For this review, take the finished solid that the model builds, in its own axes (mm). Face numbers are marked on the shaded views. A direction names the side the tool comes from. Give positions to 0.01 mm unless a question says otherwise; leave off trailing zeros. Order: outer loops, then holes, each group sorted by start corner. A loop starts at its lowest first (then second) coordinate and runs counter-clockwise, first axis right, second up.
Item 1: The part is to be moulded in two halves that separate along Y. For the marked faces 1, 2 and 3, say which applies: released by +Y, released by -Y, zero draft, split by the parting line, or undercut.
Item 2: Consider section A-A (z = -58). Give the number of separate pieces and of enclosed holes in the cut face, plus the area to 3 significant figures.
Item 3: Machinability: for the marked faces 4, 5 and 6, which of the approach directions +Z, -Z, +X, -X, +Y, -Y give a long, thin tool a straight path to every point of the face, cutting with its end or side? Answer none if there is none.
Item 4: Consider section B-B (x = 5). Give the boundary of the cut face in (y, z).
Item 5: For probe 1 along Y at (x, z) = (1.5, -26.5); probe 2 along Y at (x, z) = (-23, -48); probe 3 along Y at (x, z) = (18, -7), list the stretches that pass through material, from the lowest coordinate up.
Item 6: For P1, Ø1.2, axis at y = -24.5, z = -34, coming from the -X side; P2, Ø3, axis at y = -7, z = -25.5, coming from the -X side; P3, Ø2.5, axis at x = 13.97, y = 52.14, coming from the -Z side; P4, Ø4, axis at x = 37, z = -62, coming from the -Y side, all flat-tipped, find the tip position at first contact; note any pin that passes through.
```python
from build123d import *

# Parameters (mm, degrees)
SKETCH1_R                                     = 63.5
BOSS_EXTRUDE1_DEPTH                           = 6.35
BOSS_EXTRUDE2_START                           = 19.5
SKETCH1_3_R                                   = 44.45
BOSS_EXTRUDE2_DEPTH                           = 101.6
CUT_EXTRUDE1_DEPTH                            = 136.598893801
FILLET1_R                                     = 3.75
CUT_EXTRUDE2_DEPTH                            = 5
SKETCH4_R                                     = 63.5
SKETCH4_R_2                                   = 44.45
BOSS_EXTRUDE3_DEPTH                           = 15.4
CSK_FOR_8_FLAT_HEAD_MACHINE_SCREW1_AT_2_COUNT = 2
CSK_FOR_8_FLAT_HEAD_MACHINE_SCREW1_AT_2_PITCH = 53.975
CSK_FOR_8_FLAT_HEAD_MACHINE_SCREW1_AT_3_COUNT = 2
CSK_FOR_8_FLAT_HEAD_MACHINE_SCREW1_AT_3_PITCH = 93.487442339
CSK_FOR_8_FLAT_HEAD_MACHINE_SCREW1_AT_4_COUNT = 2
CSK_FOR_8_FLAT_HEAD_MACHINE_SCREW1_AT_4_PITCH = 107.95
CSK_FOR_8_FLAT_HEAD_MACHINE_SCREW1_AT_5_COUNT = 2
CSK_FOR_8_FLAT_HEAD_MACHINE_SCREW1_AT_5_PITCH = 93.487442339
CSK_FOR_8_FLAT_HEAD_MACHINE_SCREW1_AT_6_COUNT = 2
CSK_FOR_8_FLAT_HEAD_MACHINE_SCREW1_AT_6_PITCH = 53.975
CUT_EXTRUDE3_DEPTH                            = 127.047223293
SKETCH8_R                                     = 5.0856896
CUT_EXTRUDE4_DEPTH                            = 117.810059498
TAP_DRILL_FOR_M4X0_7_TAP1_D                   = 3.3
CUT_EXTRUDE5_START                            = -66.7
SKETCH12_R                                    = 44.45
SKETCH12_R_2                                  = 38.1
CUT_EXTRUDE5_DEPTH                            = 66.7


with BuildPart() as part:
    # Sketch1 → Boss-Extrude1 (new body)
    with BuildSketch(Plane.XY):
        Circle(SKETCH1_R)
    extrude(amount=BOSS_EXTRUDE1_DEPTH)

    # Sketch1<3> → Boss-Extrude2 (add)
    with BuildSketch(Plane.XY.offset(BOSS_EXTRUDE2_START)):
        Circle(SKETCH1_3_R)
    extrude(amount=-BOSS_EXTRUDE2_DEPTH)

    # Sketch2 → Cut-Extrude1 (cut, through all)
    with BuildSketch(Plane(origin=(0, 0, 19.5), x_dir=(-1, 0, 0), z_dir=(0, 0, -1))):
        Polygon((-19.65, 28.65), (-19.65, 19.65), (-28.65, 19.65), (-28.65, -19.65), (-19.65, -19.65), (-19.65, -28.65), (19.65, -28.65), (19.65, -19.65), (28.65, -19.65), (28.65, 19.65), (19.65, 19.65), (19.65, 28.65), align=None)
    extrude(amount=CUT_EXTRUDE1_DEPTH, mode=Mode.SUBTRACT)

    # Fillet1
    fillet1_edges = [part.edges().sort_by_distance(p)[0] for p in [
        (-19.65, 28.65, -31.3),
        (19.65, 28.65, -31.3),
        (19.65, 19.65, -31.3),
        (28.65, 19.65, -31.3),
        (28.65, -19.65, -31.3),
        (19.65, -19.65, -31.3),
        (19.65, -28.65, -31.3),
        (-19.65, -28.65, -31.3),
        (-19.65, -19.65, -31.3),
        (-28.65, -19.65, -31.3),
        (-28.65, 19.65, -31.3),
        (-19.65, 19.65, -31.3),
    ]]
    fillet(fillet1_edges, radius=FILLET1_R)

    # Sketch3 → Cut-Extrude2 (cut)
    with BuildSketch(Plane(origin=(0, 0, 19.5), x_dir=(-1, 0, 0), z_dir=(0, 0, -1))):
        with BuildLine():
            Line((-24.9, -28.65), (24.9, -28.65))
            ThreePointArc((24.9, -28.65), (27.551650429, -27.551650429), (28.65, -24.9))
            Line((28.65, -24.9), (28.65, 24.9))
            ThreePointArc((28.65, 24.9), (27.551650429, 27.551650429), (24.9, 28.65))
            Line((24.9, 28.65), (-24.9, 28.65))
            ThreePointArc((-24.9, 28.65), (-27.551650429, 27.551650429), (-28.65, 24.9))
            Line((-28.65, 24.9), (-28.65, -24.9))
            ThreePointArc((-28.65, -24.9), (-27.551650429, -27.551650429), (-24.9, -28.65))
        make_face()
    extrude(amount=CUT_EXTRUDE2_DEPTH, mode=Mode.SUBTRACT)

    # Sketch4 → Boss-Extrude3 (add)
    with BuildSketch(Plane(origin=(0, 0, 0), x_dir=(-1, 0, 0), z_dir=(0, 0, -1))):
        Circle(SKETCH4_R)
        with Locations(Location((0, 0, 0), (0, 0, 180))):
            Circle(SKETCH4_R_2, mode=Mode.SUBTRACT)
    extrude(amount=BOSS_EXTRUDE3_DEPTH)

    # Sketch7 → CSK for #8 Flat Head Machine Screw1 (revolve, cut)
    with BuildSketch(Plane(origin=(38.166088515, -38.166088515, -7.4), x_dir=(0, -1, 0), z_dir=(1, 0, 0))):
        Polygon((0, 0), (0, 74.7), (2.2479, 74.7), (2.2479, 3.264503502), (5.0856896, 0), align=None)
    csk_for_8_flat_head_machine_screw1 = revolve(axis=Axis((38.166088515, -38.166088515, -1.05), (0, 0, -1)), mode=Mode.SUBTRACT)

    # CSK for #8 Flat Head Machine Screw1 at 2: CSK for #8 Flat Head Machine Screw1 ×2
    with Locations(*[Vector(-0.9659258262890688, -0.25881904510251924, 0) * (i * CSK_FOR_8_FLAT_HEAD_MACHINE_SCREW1_AT_2_PITCH) for i in range(1, CSK_FOR_8_FLAT_HEAD_MACHINE_SCREW1_AT_2_COUNT)]):
        add(csk_for_8_flat_head_machine_screw1, mode=Mode.SUBTRACT)

    # CSK for #8 Flat Head Machine Screw1 at 3: CSK for #8 Flat Head Machine Screw1 ×2
    with Locations(*[Vector(-0.9659258262890679, 0.25881904510252224, 0) * (i * CSK_FOR_8_FLAT_HEAD_MACHINE_SCREW1_AT_3_PITCH) for i in range(1, CSK_FOR_8_FLAT_HEAD_MACHINE_SCREW1_AT_3_COUNT)]):
        add(csk_for_8_flat_head_machine_screw1, mode=Mode.SUBTRACT)

    # CSK for #8 Flat Head Machine Screw1 at 4: CSK for #8 Flat Head Machine Screw1 ×2
    with Locations(*[Vector(-0.7071067811865464, 0.7071067811865487, 0) * (i * CSK_FOR_8_FLAT_HEAD_MACHINE_SCREW1_AT_4_PITCH) for i in range(1, CSK_FOR_8_FLAT_HEAD_MACHINE_SCREW1_AT_4_COUNT)]):
        add(csk_for_8_flat_head_machine_screw1, mode=Mode.SUBTRACT)

    # CSK for #8 Flat Head Machine Screw1 at 5: CSK for #8 Flat Head Machine Screw1 ×2
    with Locations(*[Vector(-0.2588190451025193, 0.9659258262890688, 0) * (i * CSK_FOR_8_FLAT_HEAD_MACHINE_SCREW1_AT_5_PITCH) for i in range(1, CSK_FOR_8_FLAT_HEAD_MACHINE_SCREW1_AT_5_COUNT)]):
        add(csk_for_8_flat_head_machine_screw1, mode=Mode.SUBTRACT)

    # CSK for #8 Flat Head Machine Screw1 at 6: CSK for #8 Flat Head Machine Screw1 ×2
    with Locations(*[Vector(0.25881904510252257, 0.9659258262890679, 0) * (i * CSK_FOR_8_FLAT_HEAD_MACHINE_SCREW1_AT_6_PITCH) for i in range(1, CSK_FOR_8_FLAT_HEAD_MACHINE_SCREW1_AT_6_COUNT)]):
        add(csk_for_8_flat_head_machine_screw1, mode=Mode.SUBTRACT)

    # Sketch5 → Cut-Extrude3 (cut, through all)
    with BuildSketch(Plane.XY.offset(6.35)):
        with BuildLine():
            Line((-63.496824603, -0.635031756), (0.635031756, 63.496824603))
            ThreePointArc((0.635031756, 63.496824603), (-44.901280605, 44.901280605), (-63.496824603, -0.635031756))
        make_face()
    extrude(amount=-CUT_EXTRUDE3_DEPTH, mode=Mode.SUBTRACT)

    # Sketch8 → Cut-Extrude4 (cut, through all)
    with BuildSketch(Plane(origin=(0, 0, -7.4), x_dir=(-1, 0, 0), z_dir=(0, 0, -1))):
        with Locations((-38.166088515, -38.166088515)):
            Circle(SKETCH8_R)
        with Locations((52.135846474, -13.969757959)):
            Circle(SKETCH8_R)
        with Locations((13.969757959, -52.135846474)):
            Circle(SKETCH8_R)
        with Locations((-52.135846474, 13.969757959)):
            Circle(SKETCH8_R)
        with Locations((-13.969757959, 52.135846474)):
            Circle(SKETCH8_R)
    extrude(amount=-CUT_EXTRUDE4_DEPTH, mode=Mode.SUBTRACT)

    # Tap Drill for M4x0.7 Tap1 (through all)
    with Locations(Plane.XY.offset(14.5)):
        with Locations((-23.57, 23.57), (23.57, 23.57), (23.57, -23.57), (-23.57, -23.57)):
            Hole(TAP_DRILL_FOR_M4X0_7_TAP1_D / 2)

    # Sketch12 → Cut-Extrude5 (cut)
    with BuildSketch(Plane(origin=(0, 0, -82.1), x_dir=(-1, 0, 0), z_dir=(0, 0, -1)).offset(CUT_EXTRUDE5_START)):
        with Locations(Location((0, 0, 0), (0, 0, 180))):
            Circle(SKETCH12_R)
        Circle(SKETCH12_R_2, mode=Mode.SUBTRACT)
    extrude(amount=CUT_EXTRUDE5_DEPTH, mode=Mode.SUBTRACT)


solid = part.part
```
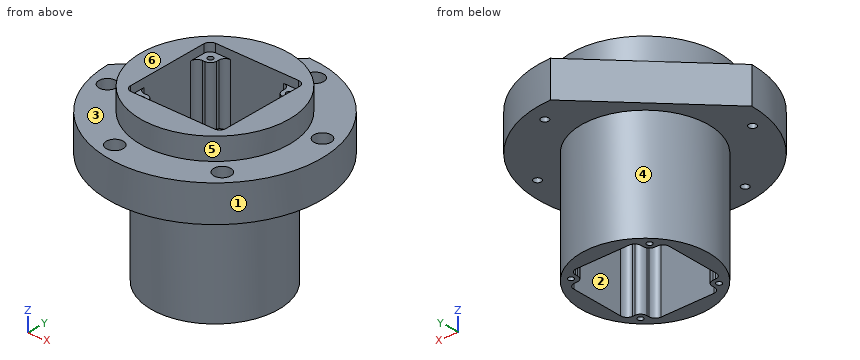
Resolved:
1. face 1: split by the parting line
1. face 2: undercut
1. face 3: zero draft
2. separate pieces: 1
2. enclosed holes: 5
2. area: 1,580 mm2
3. face 4: -Z
3. face 5: +Z
3. face 6: +Z, +X, -X, +Y, -Y
4. outline: (-63.3, -15.4) - (-37.77, -15.4) - (-37.77, -82.1) - (-28.65, -82.1) - (-28.65, 19.5) - (-44.17, 19.5) - (-44.17, 6.35) - (-63.3, 6.35) - close; (28.65, -82.1) - (37.77, -82.1) - (37.77, -15.4) - (63.3, -15.4) - (63.3, 6.35) - (44.17, 6.35) - (44.17, 19.5) - (28.65, 19.5) - close
5. probe 1: y = -38.07 to -28.65, 28.65 to 38.07
5. probe 2: y = -30.37 to -25.12, -22.02 to -19.67, 19.67 to 22.02, 25.12 to 30.37
5. probe 3: y = -60.9 to -28.01, 28.01 to 49.03, 55.24 to 60.9
6. P1: stops at x = -29.67
6. P2: stops at x = -37.7
6. P3: passes through
6. P4: stops at y = -15.05
